The model under review builds one solid part; all positions refer to its coordinate system, in mm. A direction names the side the tool comes from. Round coordinates to 2 decimals unless told otherwise and drop trailing zeros. Loops run counter-clockwise (first coordinate to the right, second up) from the corner with the lowest first, then second, coordinate; pieces in that order, holes last. Notation, with made-up numbers: M 85.5,6 L 140.5,6 A23 ccw 140.5,15 Z; hole C 13,60.25 d11. An arc over 180 degrees is marked long. Return JSON: item names as keys, results as strings. Group by question number.
Q1. Consider section A-A (z = 71). State the section outline as (x, y) points, and give its area (3 significant figures).
Q2. Consider section B-B (x = 322). Count the separate pieces of the cut face and the enclosed holes in it, and give its area (3 significant figures).
Q3. Clearance check with flat-ended pins moving along their axes: pin 1 Ø3 at (x, z) = (62.5, 344.5) entering from +Y; pin 2 Ø11.5 at (x, y) = (135, 25) entering from -Z; pin 3 Ø8 at (x, z) = (350.5, 303.5) entering from -Y. State where each tip first meets the part, or that it passes through.
Q4. To check wall thickness, follow line 1 along X through (y, z) = (29, 146); line 2 along Y through (x, z) = (330, 153); line 3 along X through (y, z) = (45, 386.5) (3 decimals). State the ranges of each line that lie inside material, in increasing order.
Q5. Draft analysis for pull direction X (two halves, no side actions). For faces 6 (the face through (201, 6, 279.4)), 7 (the face through (201, 368.3, 138)), 8 (the face through (215, 374, 406.4)), 9 (the face through (406.4, 200, 150)), state which applies: pulls with the +X half, pulls with the -X half, needs draft (parallel to the pull), parting line crosses it, or undercut.
Q6. For faces 1 (the face through (201, 12.7, 138)), 2 (the face through (201, 19, 304.8)), 3 (the face through (201, 368.3, 355)), 4 (the face through (172, 370, 0)), 5 (the face through (0, 200, 150)), list the 3-axis set-ups (+Z, -Z, +X, -X, +Y, -Y) from which the entire face can be reached by the end or side of a thin tool; tool diameter is ignored.
from build123d import *

# Parameters (mm, degrees)
SKETCH1_W               = 406.4
SKETCH1_H               = 406.4
BOSS_EXTRUDE1_DEPTH     = 304.8
CUT_EXTRUDE2_DEPTH      = 704.905448311
CUT_EXTRUDE2_DEPTH_BACK = 704.905448311
SKETCH6_W               = 330.2
SKETCH6_H               = 330.2
CUT_EXTRUDE3_DEPTH      = 704.905448369
CUT_EXTRUDE3_DEPTH_BACK = 704.905448369
SKETCH7_W               = 330.2
SKETCH7_H               = 25.4
SKETCH8_W               = 330.2
SKETCH8_H               = 279.4
CUT_EXTRUDE4_DEPTH      = 25.4


with BuildPart() as part:
    # Sketch1 → Boss-Extrude1 (new body)
    with BuildSketch(Plane.XY):
        with Locations((203.2, 203.2)):
            Rectangle(SKETCH1_W, SKETCH1_H)
    extrude(amount=BOSS_EXTRUDE1_DEPTH)

    # Sketch2 → section 1 of loft1
    with BuildSketch(Plane.XY.offset(406.4), mode=Mode.PRIVATE) as loft1_s1:
        with BuildLine():
            Line((25.4, 25.4), (381, 25.4))
            Line((381, 25.4), (381, 381))
            Line((381, 381), (25.4, 381))
            Line((25.4, 381), (25.4, 25.4))
        make_face()
    # loft from a face of the part (loft1)
    loft([part.faces().sort_by_distance((203.2, 203.2, 304.8))[0], loft1_s1.sketch])

    # Sketch6 → Cut-Extrude2 (cut, two sides: drawn at the far end of the back side and taken through both)
    with BuildSketch(Plane.XY.offset(406.4).offset(-CUT_EXTRUDE2_DEPTH_BACK)):
        with Locations((203.2, 203.2)):
            Rectangle(SKETCH6_W, SKETCH6_H)
    extrude(amount=CUT_EXTRUDE2_DEPTH + CUT_EXTRUDE2_DEPTH_BACK, mode=Mode.SUBTRACT)

    # Sketch7 → Cut-Extrude3 (cut, two sides: drawn at the far end of the back side and taken through both)
    with BuildSketch(Plane(origin=(0, 406.4, 0), x_dir=(1, 0, 0), z_dir=(0, 1, 0)).offset(-CUT_EXTRUDE3_DEPTH_BACK)):
        with Locations((203.2, -292.1)):
            Rectangle(SKETCH7_W, SKETCH7_H)
    extrude(amount=CUT_EXTRUDE3_DEPTH + CUT_EXTRUDE3_DEPTH_BACK, mode=Mode.SUBTRACT)

    # Sketch8 → Cut-Extrude4 (cut)
    with BuildSketch(Plane(origin=(0, 38.1, 0), x_dir=(1, 0, 0), z_dir=(0, 1, 0))):
        with Locations((203.2, -139.7)):
            Rectangle(SKETCH8_W, SKETCH8_H)
    extrude(amount=-CUT_EXTRUDE4_DEPTH, mode=Mode.SUBTRACT)


solid = part.part
Values:
{
 "1": {"outline": "M 0,0 L 406.4,0 L 406.4,406.4 L 0,406.4 Z; hole M 38.1,12.7 L 368.3,12.7 L 368.3,368.3 L 38.1,368.3 Z", "area": "47,700 mm2"},
 "2": {"separate pieces": "4", "enclosed holes": "0", "area": "19,400 mm2"},
 "3": {"pin 1": "stops at y = 396.85", "pin 2": "stops at z = 304.8", "pin 3": "stops at y = 0"},
 "4": {"line 1": "x = 0 to 38.1, 368.3 to 406.4", "line 2": "y = 0 to 12.7, 368.3 to 406.4", "line 3": "x = 20.425 to 38.1, 368.3 to 385.975"},
 "5": {"face 6": "undercut", "face 7": "undercut", "face 8": "needs draft", "face 9": "pulls with the +X half"},
 "6": {"face 1": "-Z", "face 2": "+Y, -Y", "face 3": "+Z, -Z", "face 4": "-Z, +X, -X, +Y, -Y", "face 5": "+Z, -Z, -X, +Y, -Y"}
}
